Input: dimensioned drawing with shaded views. Units: mm. Origin: part minimum x, y, z. A direction names the side the tool comes from. Give positions to 0.01 mm unless a question says otherwise; leave off trailing zeros. Write each loop counter-clockwise with the first axis right and the second up, starting at its lowest first coordinate (ties: lowest second). Pieces come first, ordered by that corner, then holes. Notation, with made-up numbers: M 63.25,-12 L 87.25,-12 A23 ccw 87.25,11 Z; hole C 0.25,77 d10. An arc over 180 degrees is marked long. Answer as a JSON object with one key per item and string values.
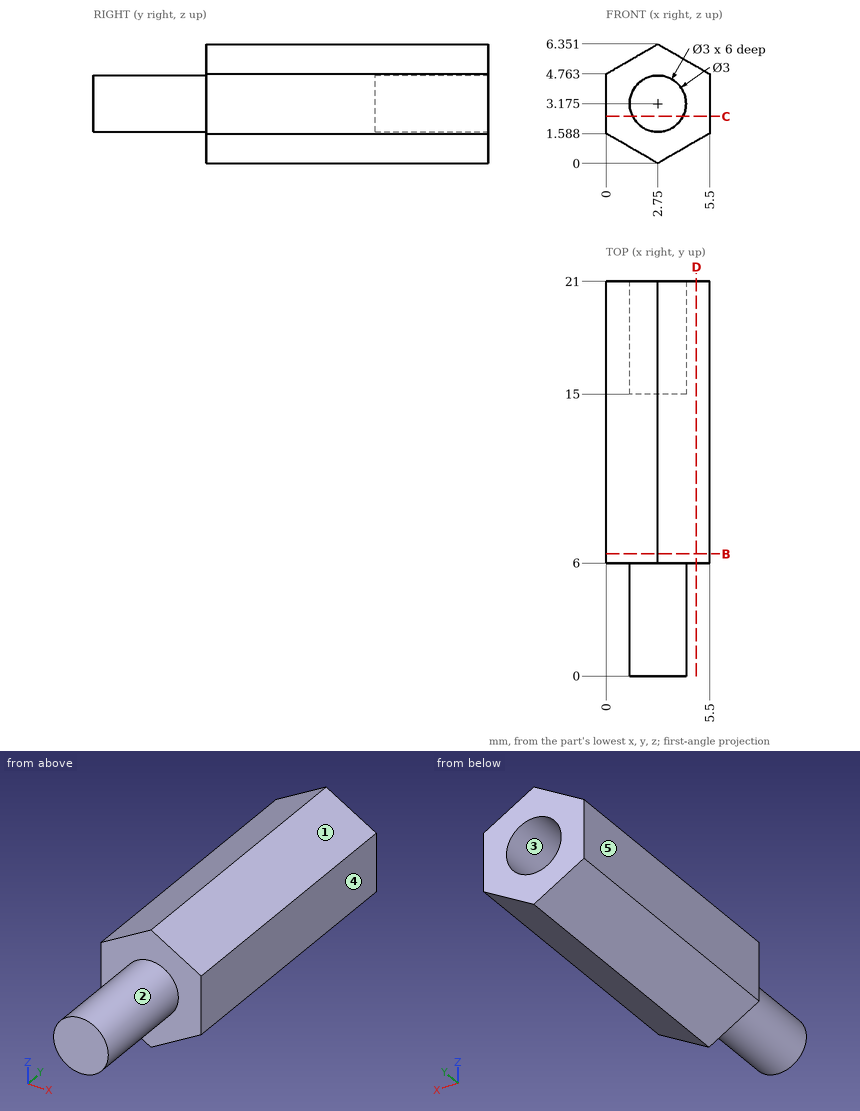
1) Line query: line 1 (Y direction, x = 2.2, z = 5); line 2 (X direction, y = 4.75, z = 3.25); line 3 (Y direction, x = 2, z = 3.75). Output: solid intervals per line, ascending. Write a range as from..to.
Geometry check:
{"line 1": "y = 6..21", "line 2": "x = 1.25..4.25", "line 3": "y = 0..15"}
2) Cut plane D-D on x = 4.8. Return loops of the section in (y, z).
Geometry check:
{"outline": "M 6,1.18 L 21,1.18 L 21,5.17 L 6,5.17 Z"}
3) Set-up query: the marked faces 1 and 2. Return all of +Z, -Z, +X, -X, +Y, -Y with unobstructed straight access to the full face (end or side cutting, diameter ignored); none if empty.
Geometry check:
{"face 1": "+Z, +X, +Y, -Y", "face 2": "-Y"}
4) Cut plane C-C on z = 2.5. Return loops of the section in (x, y).
Geometry check:
{"outline": "M 0,6 L 1.41,6 L 1.41,0 L 4.09,0 L 4.09,6 L 5.5,6 L 5.5,21 L 4.09,21 L 4.09,15 L 1.41,15 L 1.41,21 L 0,21 Z"}
5) Cut plane B-B on y = 6.5. Return loops of the section in (x, z), and give its area (3 significant figures).
Geometry check:
{"outline": "M 0,1.59 L 2.75,0 L 5.5,1.59 L 5.5,4.76 L 2.75,6.35 L 0,4.76 Z", "area": "26.2 mm2"}
6) Pull-direction query (X, two-part tool) for the marked faces 3, 4 and 5; classes: pulls with the +X half, pulls with the -X half, needs draft (parallel to the pull), parting line crosses it, or undercut.
Geometry check:
{"face 3": "undercut", "face 4": "pulls with the +X half", "face 5": "pulls with the -X half"}
7) Contact query for flat-ended pins moving along their axis: P1, Ø0.9, axis at x = 2.5, z = 3, coming from the +Y side; P2, Ø3, axis at x = 3, z = 3.5, coming from the -Y side. Output: stop coordinate, or through.
Geometry check:
{"P1": "stops at y = 15", "P2": "stops at y = 0"}
